Build history of the part. All positions in model axes, mm. A direction names the side the tool comes from. Round coordinates to 2 decimals unless told otherwise and drop trailing zeros. Order: outer loops, then holes, each group sorted by start corner. A loop starts at its lowest first (then second) coordinate and runs counter-clockwise, first axis right, second up. Notation, with made-up numbers: (69, 82) -> (84, 82) arc R25 ccw to (84, 119) -> close; hole circle Ø11 at (67, -8.5). An arc over 180 degrees is marked (long way). Answer as a JSON object with one key per item and string values.
Autodesk Inventor part; units mm, degrees
ref_plane "YZ Plane" through (0, 0, 0) normal (1, 0, 0) x (0, 1, 0)
ref_plane "XZ Plane" through (0, 0, 0) normal (0, 1, 0) x (-1, 0, 0)
ref_plane "XY Plane" through (0, 0, 0) normal (0, 0, 1) x (1, 0, 0)
sketch "Esboço3" plane through (0, 0, 0) normal (0, 1, 0) x (-1, 0, 0)
  line L0 (0, 0) -> (70, 0)
  line L1 (70, 0) -> (70, -50)
  line L2 (70, -50) -> (0, -50)
  line L3 (0, -50) -> (0, 0)
  dimension "d4" = 70
  dimension "d5" = 50
extrude "Extrusão2" add sketch "Esboço3" along normal blind 0.2
sketch "Esboço4" plane through (0, 0.2, 0) normal (0, 1, 0) x (1, 0, 0)
  line L0 (0, 0) -> (0, 50)
  line L1 (0, 50) -> (-45, 50)
  line L2 (-45, 50) -> (-45, 48)
  line L3 (-45, 48) -> (0, 48)
  line L4 (0, 48) -> (0, 50)
  line L5 (-70, 0) -> (0, 0)
  line L6 (0, 0) -> (-37.5, 0)
  line L7 (-37.5, 0) -> (-37.5, 2)
  line L8 (-37.5, 2) -> (0, 2)
  line L9 (0, 2) -> (0, 0)
  line L10 (0, 2) -> (0, 12)
  line L11 (0, 12) -> (-33, 12)
  line L12 (-33, 12) -> (-33, 22)
  line L13 (-33, 22) -> (0, 22)
  line L14 (0, 22) -> (0, 12)
  dimension "d8" = 45
  dimension "d9" = 2
  dimension "d10" = 37.5
  dimension "d11" = 2
  dimension "d12" = 10
  dimension "d13" = 33
  dimension "d14" = 10
extrude "Extrusão3" add sketch "Esboço4" along normal blind 10
sketch "Esboço5" plane through (0, 0.2, 0) normal (0, 1, 0) x (1, 0, 0)
  line L0 (-70, 0) -> (-70, 2.1)
  line L1 (-70, 50) -> (-70, 0)
  line L2 (-70, 2.1) -> (-60, 2.1)
  line L3 (-60, 2.1) -> (-60, 12.1)
  line L4 (-60, 12.1) -> (-72, 12.1)
  line L5 (-60, 2.1) -> (-72, 2.1)
  line L6 (-72, 2.1) -> (-72, 12.1)
  line L7 (-72, 12.1) -> (-60, 12.1)
  line L8 (-60, 12.1) -> (-60, 2.1)
  point P0 (0, 0)
  point P1 (-70, 12.1)
extrude "Extrusão4" add sketch "Esboço5" along normal blind 10 contours L4 L3 L2 L1
sketch "Esboço7" plane through (-70, 0, -50) normal (-1, 0, 0) x (0, 0, 1)
  line L0 (48, 0.2) -> (48, 10.2)
  line L1 (48, 0.2) -> (38, 0.2)
  line L2 (48, 10.2) -> (38, 10.2)
  line L3 (38, 10.2) -> (38, 0.2)
  line L4 (38, 0.2) -> (48, 0.2)
  line L5 (48, 0.2) -> (48, 10.2)
  point P0 (50, 0)
extrude "Extrusão5" add sketch "Esboço7" along normal blind 2
sketch "Esboço8" plane through (0, 0.2, 0) normal (0, 1, 0) x (1, 0, 0)
  line L0 (-60, 12.1) -> (-70, 12.1)
  line L1 (-70, 12.1) -> (-70, 32.1)
  line L2 (-70, 50) -> (-70, 12.1)
  line L3 (-70, 32.1) -> (-70, 39.6)
  line L4 (-70, 32.1) -> (-60, 32.1)
  line L5 (-60, 32.1) -> (-60, 42.1)
  line L6 (-60, 42.1) -> (-70, 42.1)
  line L7 (-70, 42.1) -> (-70, 32.1)
  point P0 (0, 0)
extrude "Extrusão6" add sketch "Esboço8" along normal blind 10
sketch "Esboço9" plane through (-70, 0, -50) normal (-1, 0, 0) x (0, 0, 1)
  line L0 (17.9, 10.2) -> (7.9, 10.2)
  line L1 (7.9, 10.2) -> (7.9, 0.2)
  line L2 (7.9, 0.2) -> (17.9, 0.2)
  line L3 (17.9, 0.2) -> (17.9, 10.2)
  point P0 (50, 0)
  dimension "d32" = 10
  dimension "d33" = 10
extrude "Extrusão7" add sketch "Esboço9" along normal blind 5
properties part number "arduinoUNO"
1) Which spindle directions (+Z, -Z, +X, -X, +Y, -Y) get a long thin tool onto all of the face, cutting with end or side? Do faces 4 (the face through (-72, 5, -7)), 5 (the face through (-71, 0.2, -7)), 6 (the face through (-17, 5, -22)). Say none if no direction does.
Checked values:
{"face 4": "+Z, -X, +Y, -Y", "face 5": "+Z, -Z, -X, -Y", "face 6": "+X, -X, +Y"}
2) Pull direction Z, two halves, no side cores. Call faces 1 (the face through (-19, 5, 0)), 2 (the face through (-35, 0.2, -25)), 3 (the face through (-23, 10.2, -49)): pulls with the +Z half, pulls with the -Z half, needs draft (parallel to the pull), parting line crosses it, or undercut.
Checked values:
{"face 1": "pulls with the +Z half", "face 2": "undercut", "face 3": "needs draft"}
3) Cut at D-D, the plane z = -18. Give the cut face in (x, y).
Checked values:
{"outline": "(-70, 0) -> (0, 0) -> (0, 10.2) -> (-33, 10.2) -> (-33, 0.2) -> (-70, 0.2) -> close"}
4) Probe L1, parallel to Z at x = -15, y = 9.5; L2, parallel to Z at x = -68.5, y = 4.25; L3, parallel to Z at x = -37, y = 6. List the from-to ranges inside material, lowest first. Write a range as from..to.
Checked values:
{"L1": "z = -50..-48, -22..-12, -2..0", "L2": "z = -42.1..-32.1, -12.1..-2.1", "L3": "z = -50..-48, -2..0"}
5) Flat gauge pins, fed straight in: pin 1 Ø2 at (y, z) = (5, -49) entering from -X; pin 2 Ø1.6 at (x, y) = (-71, 3.5) entering from -Z; pin 3 Ø2 at (x, y) = (-61.5, 7) entering from +Z. Where does each tip first touch, or does it go through?
Checked values:
{"pin 1": "stops at x = -45", "pin 2": "stops at z = -42.1", "pin 3": "stops at z = -2.1"}
6) Cut at B-B, the plane z = -35.5. Give the cut face in (x, y), plus the area to 3 significant figures.
Checked values:
{"outline": "(-75, 0.2) -> (-70, 0.2) -> (-70, 0) -> (0, 0) -> (0, 0.2) -> (-60, 0.2) -> (-60, 10.2) -> (-75, 10.2) -> close", "area": "164 mm²"}
7) Cut at C-C, the plane x = -7.5. Give the cut face in (y, z).
Checked values:
{"outline": "(0, -50) -> (10.2, -50) -> (10.2, -48) -> (0.2, -48) -> (0.2, -22) -> (10.2, -22) -> (10.2, -12) -> (0.2, -12) -> (0.2, -2) -> (10.2, -2) -> (10.2, 0) -> (0, 0) -> close"}
8) Cut at A-A, the plane y = 6.5. Give the cut face in (x, z).
Checked values:
{"outline": "(-75, -42.1) -> (-60, -42.1) -> (-60, -32.1) -> (-75, -32.1) -> close; (-72, -12) -> (-70, -12) -> (-70, -12.1) -> (-60, -12.1) -> (-60, -2.1) -> (-70, -2.1) -> (-70, -2) -> (-72, -2) -> close; (-45, -50) -> (0, -50) -> (0, -48) -> (-45, -48) -> close; (-37.5, -2) -> (0, -2) -> (0, 0) -> (-37.5, 0) -> close; (-33, -22) -> (0, -22) -> (0, -12) -> (-33, -12) -> close"}
